For this review, use the dimensioned drawing (mm, ordinates from the lowest corner) and the shaded views. A direction names the side the tool comes from. Coordinates: 2 decimals unless noted, no trailing zeros. Loops run counter-clockwise (first coordinate to the right, second up) from the corner with the lowest first, then second, coordinate; pieces in that order, holes last. Notation, with made-up numbers: M 24,38 L 82,38 A23 ccw 82,68 Z; hole C 59,13.5 d6. An arc over 180 degrees is marked long. One line per item, written item: value.
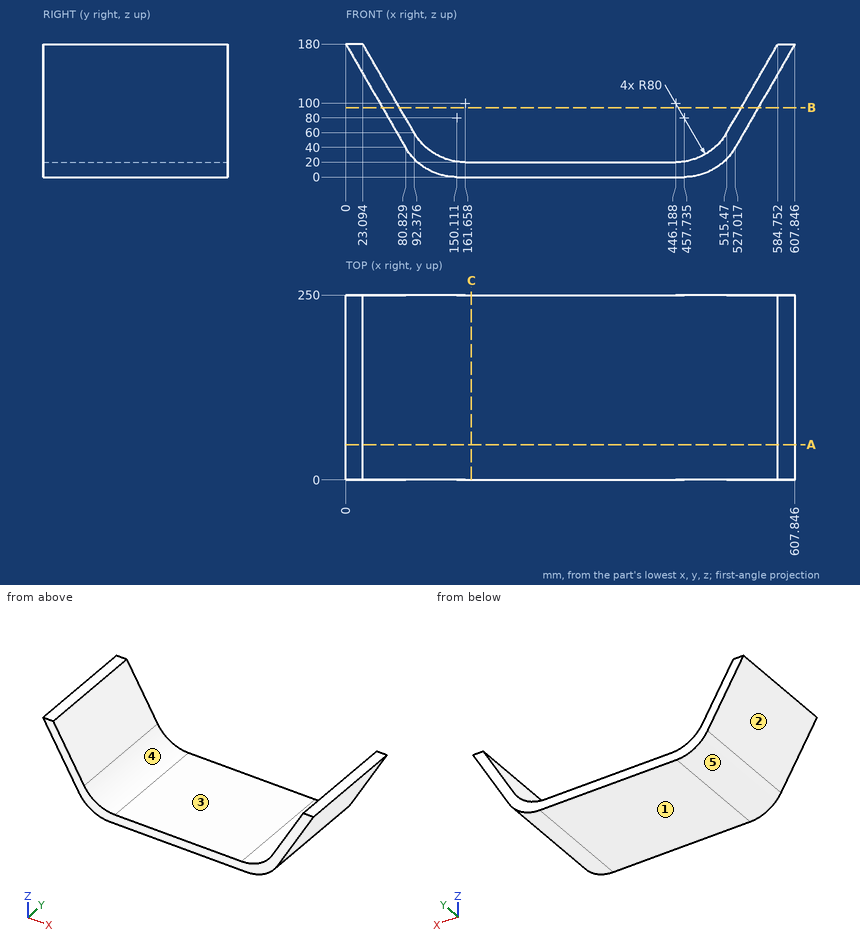
(1) To check wall thickness, follow L1, parallel to Z at x = 185, y = 117; L2, parallel to X at y = 65, z = 76; L3, parallel to X at y = 220, z = 168. State the ranges of each line that lie inside material, in increasing order. Write a range as [from, to].
Checks:
L1: [0, 20]
L2: [60.04, 83.14], [524.71, 547.8]
L3: [6.93, 30.02], [577.82, 600.92]
(2) Add section B-B on z = 94. State the section outline as (x, y) points.
Checks:
outline: M 49.65,0 L 72.75,0 L 72.75,250 L 49.65,250 Z; M 535.1,0 L 558.19,0 L 558.19,250 L 535.1,250 Z
(3) Insertion check: pin 1 Ø3 at (y, z) = (165, 48.5) entering from -X; pin 2 Ø3 at (y, z) = (175.5, 66.5) entering from +X; pin 3 Ø6 at (x, y) = (470.5, 117) entering from +Z. Each pin has a flat end and moves straight along its axis. Give the tip position at first contact, or say it passes through.
Checks:
pin 1: x = 75.06
pin 2: x = 543.18
pin 3: z = 24.81
(4) Tool access review of the marked faces 4 and 5: name each direction out of +Z, -Z, +X, -X, +Y, -Y from which nothing blocks a thin tool from reaching the whole face with its end or side.
Checks:
face 4: +Z, +Y, -Y
face 5: -Z, -X, +Y, -Y
(5) Draft analysis for pull direction X (two halves, no side actions). For the marked faces 1, 2 and 3, state which applies: pulls with the +X half, pulls with the -X half, needs draft (parallel to the pull), parting line crosses it, or undercut.
Checks:
face 1: needs draft
face 2: pulls with the -X half
face 3: undercut
(6) Add section A-A on y = 47.5. State the section outline as (x, z) points (3 decimals), then the cut area to 3 significant figures.
Checks:
outline: M 0,180 L 80.829,40 A80 ccw 150.111,0 L 457.735,0 A80 ccw 527.017,40 L 607.846,180 L 584.752,180 L 515.47,60 A80 cw 446.188,20 L 161.658,20 A80 cw 92.376,60 L 23.094,180 Z
area: 15,600 mm^2
(7) Add section C-C on x = 170. State the section outline as (y, z) points.
Checks:
outline: M 0,0 L 250,0 L 250,20 L 0,20 Z
